Check sheet for the drawn part. Datum: minimum x, y, z corner. Units: mm. Round coordinates to 2 decimals unless told otherwise and drop trailing zeros. Write each loop counter-clockwise with the first axis right and the second up, starting at its lowest first coordinate (ties: lowest second). Pieces come first, ordered by that corner, then holes. Notation, with made-up numbers: M 4.5,46.5 L 62.5,46.5 A19 cw 62.5,71.5 Z; hole C 19,35 d5. An arc over 180 degrees is marked long. Use a Markdown table: item, result.
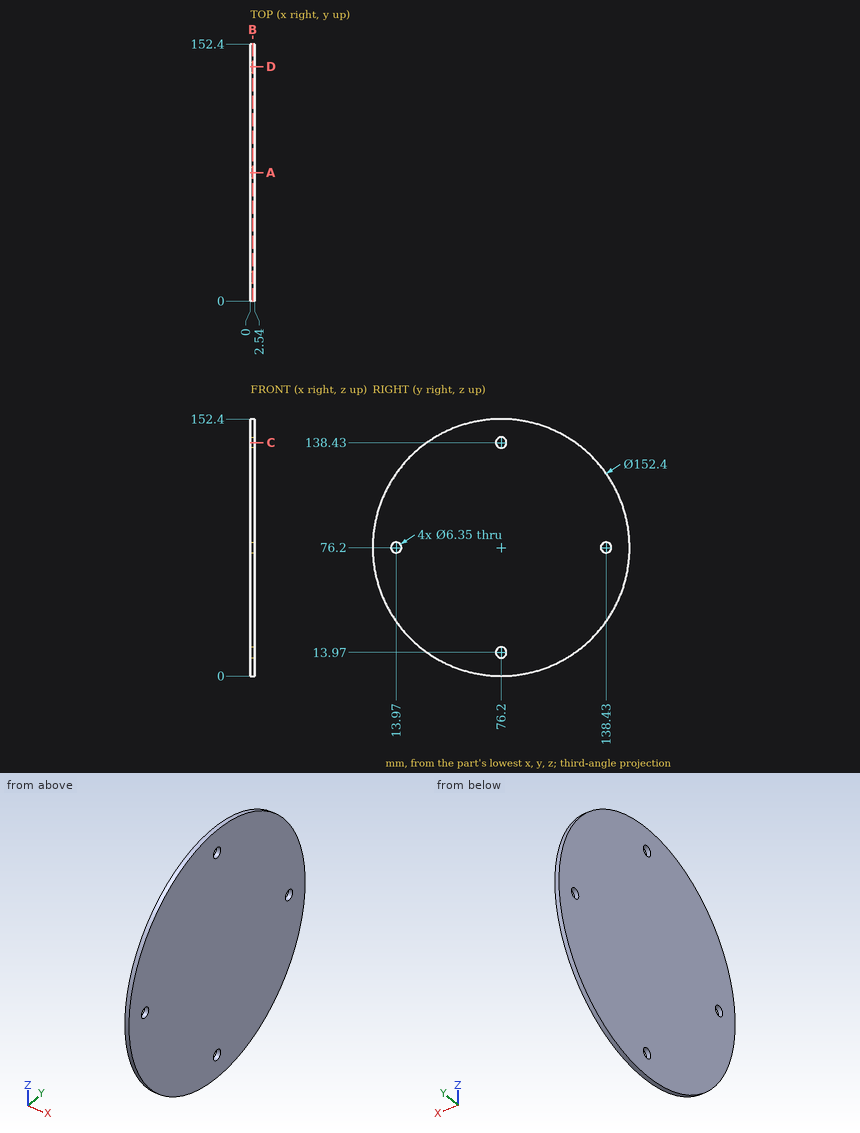
Item 1: Cross-section at D-D, the plane y = 139. Record the cut outline in (x, z).
Outcome:
| item | result |
|---|---|
| outline | M 0,33.04 L 2.54,33.04 L 2.54,73.08 L 0,73.08 Z; M 0,79.32 L 2.54,79.32 L 2.54,119.36 L 0,119.36 Z |
Item 2: Cross-section at A-A, the plane y = 76.2. Record the cut outline in (x, z) (3 decimals), and give its area (3 significant figures).
Outcome:
| item | result |
|---|---|
| outline | M 0,0 L 2.54,0 L 2.54,10.795 L 0,10.795 Z; M 0,17.145 L 2.54,17.145 L 2.54,135.255 L 0,135.255 Z; M 0,141.605 L 2.54,141.605 L 2.54,152.4 L 0,152.4 Z |
| area | 355 mm2 |
Item 3: Cross-section at B-B, the plane x = 1.35. Record the cut outline in (y, z) (3 decimals).
Outcome:
| item | result |
|---|---|
| outline | C 76.2,76.2 d152.4; hole C 13.97,76.2 d6.35; hole C 76.2,13.97 d6.35; hole C 76.2,138.43 d6.35; hole C 138.43,76.2 d6.35 |
Item 4: Cross-section at C-C, the plane z = 138.43. Record the cut outline in (x, y) (3 decimals).
Outcome:
| item | result |
|---|---|
| outline | M 0,32.224 L 2.54,32.224 L 2.54,73.025 L 0,73.025 Z; M 0,79.375 L 2.54,79.375 L 2.54,120.176 L 0,120.176 Z |
Item 5: Material ranges on line 1 along Z through (x, y) = (1.7, 13.97) (3 decimals); line 2 along Z through (x, y) = (0.1, 135), recorded low to high. Write a range as from..to.
Outcome:
| item | result |
|---|---|
| line 1 | z = 32.224..73.025, 79.375..120.176 |
| line 2 | z = 27.73..124.67 |
Item 6: Go/stop test with a flat-tipped pin: pin 1 (1 mm diameter, centred on x = 2, z = 107.5, fed in from +Y). Record where the tip stops, or that it passes through.
Outcome:
| item | result |
|---|---|
| pin 1 | stops at y = 145.9 |
